Design review of the part built by this model. Coordinates are the model's own, in mm. A direction names the side the tool comes from. Round coordinates to 2 decimals unless told otherwise and drop trailing zeros. Loops run counter-clockwise (first coordinate to the right, second up) from the corner with the lowest first, then second, coordinate; pieces in that order, holes last. Notation, with made-up numbers: (10, 20) - (30, 20) arc R34 cw to (30, 50) - close; hole circle Ø9 at (-36, 42.25). An arc over 180 degrees is marked (long way). Return JSON: item names as keys, results as strings. Group by question number.
from build123d import *

# Parameters (mm, degrees)
SKETCH_1_W          = 50
SKETCH_1_H          = 13
SKETCH_1_R          = 0.5
EXTRUDE_1_DEPTH     = 1.5
SKETCH_3_W          = 7.25
SKETCH_3_H          = 5
EXTRUDE_2_DEPTH     = 4
SKETCH_4_W          = 7.25
SKETCH_4_H          = 5.5
EXTRUDE_3_DEPTH     = 3
CUT_EXTRUDE_1_DEPTH = 7.25
SKETCH_6_W          = 4.302717404
SKETCH_6_H          = 3.6
SKETCH_6_W_2        = 3.2
SKETCH_6_H_2        = 1.274490689
CUT_EXTRUDE_2_DEPTH = 5


with BuildPart() as part:
    # Эскиз1 → Бобышка-Вытянуть1 (new body)
    with BuildSketch(Plane(origin=(0, 0, 0), x_dir=(1, 0, 0), z_dir=(0, 1, 0))):
        with Locations((25, 6.5)):
            Rectangle(SKETCH_1_W, SKETCH_1_H)
        with Locations(Location((1.25, 12, 0), (0, 0, 270))):
            Circle(SKETCH_1_R, mode=Mode.SUBTRACT)
        with Locations(Location((3.75, 12, 0), (0, 0, 270))):
            Circle(SKETCH_1_R, mode=Mode.SUBTRACT)
        with Locations(Location((6.25, 12, 0), (0, 0, 270))):
            Circle(SKETCH_1_R, mode=Mode.SUBTRACT)
        with Locations(Location((8.75, 12, 0), (0, 0, 270))):
            Circle(SKETCH_1_R, mode=Mode.SUBTRACT)
        with Locations(Location((11.25, 12, 0), (0, 0, 270))):
            Circle(SKETCH_1_R, mode=Mode.SUBTRACT)
        with Locations(Location((13.75, 12, 0), (0, 0, 270))):
            Circle(SKETCH_1_R, mode=Mode.SUBTRACT)
        with Locations(Location((16.25, 12, 0), (0, 0, 270))):
            Circle(SKETCH_1_R, mode=Mode.SUBTRACT)
        with Locations(Location((18.75, 12, 0), (0, 0, 270))):
            Circle(SKETCH_1_R, mode=Mode.SUBTRACT)
        with Locations(Location((21.25, 12, 0), (0, 0, 270))):
            Circle(SKETCH_1_R, mode=Mode.SUBTRACT)
        with Locations(Location((23.75, 12, 0), (0, 0, 270))):
            Circle(SKETCH_1_R, mode=Mode.SUBTRACT)
        with Locations(Location((26.25, 12, 0), (0, 0, 270))):
            Circle(SKETCH_1_R, mode=Mode.SUBTRACT)
        with Locations(Location((28.75, 12, 0), (0, 0, 270))):
            Circle(SKETCH_1_R, mode=Mode.SUBTRACT)
        with Locations(Location((31.25, 12, 0), (0, 0, 270))):
            Circle(SKETCH_1_R, mode=Mode.SUBTRACT)
        with Locations(Location((33.75, 12, 0), (0, 0, 270))):
            Circle(SKETCH_1_R, mode=Mode.SUBTRACT)
        with Locations(Location((36.25, 12, 0), (0, 0, 270))):
            Circle(SKETCH_1_R, mode=Mode.SUBTRACT)
        with Locations(Location((3.75, 1, 0), (0, 0, 270))):
            Circle(SKETCH_1_R, mode=Mode.SUBTRACT)
        with Locations(Location((6.25, 1, 0), (0, 0, 270))):
            Circle(SKETCH_1_R, mode=Mode.SUBTRACT)
        with Locations(Location((8.75, 1, 0), (0, 0, 270))):
            Circle(SKETCH_1_R, mode=Mode.SUBTRACT)
        with Locations(Location((11.25, 1, 0), (0, 0, 270))):
            Circle(SKETCH_1_R, mode=Mode.SUBTRACT)
        with Locations(Location((13.75, 1, 0), (0, 0, 270))):
            Circle(SKETCH_1_R, mode=Mode.SUBTRACT)
        with Locations(Location((16.25, 1, 0), (0, 0, 270))):
            Circle(SKETCH_1_R, mode=Mode.SUBTRACT)
        with Locations(Location((18.75, 1, 0), (0, 0, 270))):
            Circle(SKETCH_1_R, mode=Mode.SUBTRACT)
        with Locations(Location((21.25, 1, 0), (0, 0, 270))):
            Circle(SKETCH_1_R, mode=Mode.SUBTRACT)
        with Locations(Location((23.75, 1, 0), (0, 0, 270))):
            Circle(SKETCH_1_R, mode=Mode.SUBTRACT)
        with Locations(Location((26.25, 1, 0), (0, 0, 270))):
            Circle(SKETCH_1_R, mode=Mode.SUBTRACT)
        with Locations(Location((28.75, 1, 0), (0, 0, 270))):
            Circle(SKETCH_1_R, mode=Mode.SUBTRACT)
        with Locations(Location((31.25, 1, 0), (0, 0, 270))):
            Circle(SKETCH_1_R, mode=Mode.SUBTRACT)
        with Locations(Location((33.75, 1, 0), (0, 0, 270))):
            Circle(SKETCH_1_R, mode=Mode.SUBTRACT)
        with Locations(Location((36.25, 1, 0), (0, 0, 270))):
            Circle(SKETCH_1_R, mode=Mode.SUBTRACT)
        with Locations(Location((1.25, 1, 0), (0, 0, 270))):
            Circle(SKETCH_1_R, mode=Mode.SUBTRACT)
        with Locations(Location((38.75, 12, 0), (0, 0, 270))):
            Circle(SKETCH_1_R, mode=Mode.SUBTRACT)
        with Locations(Location((41.25, 12, 0), (0, 0, 270))):
            Circle(SKETCH_1_R, mode=Mode.SUBTRACT)
        with Locations(Location((43.75, 12, 0), (0, 0, 270))):
            Circle(SKETCH_1_R, mode=Mode.SUBTRACT)
        with Locations(Location((46.25, 12, 0), (0, 0, 270))):
            Circle(SKETCH_1_R, mode=Mode.SUBTRACT)
        with Locations(Location((48.75, 12, 0), (0, 0, 270))):
            Circle(SKETCH_1_R, mode=Mode.SUBTRACT)
        with Locations(Location((38.75, 1, 0), (0, 0, 270))):
            Circle(SKETCH_1_R, mode=Mode.SUBTRACT)
        with Locations(Location((41.25, 1, 0), (0, 0, 270))):
            Circle(SKETCH_1_R, mode=Mode.SUBTRACT)
        with Locations(Location((43.75, 1, 0), (0, 0, 270))):
            Circle(SKETCH_1_R, mode=Mode.SUBTRACT)
        with Locations(Location((46.25, 1, 0), (0, 0, 270))):
            Circle(SKETCH_1_R, mode=Mode.SUBTRACT)
        with Locations(Location((48.75, 1, 0), (0, 0, 270))):
            Circle(SKETCH_1_R, mode=Mode.SUBTRACT)
    extrude(amount=EXTRUDE_1_DEPTH)

    # Эскиз3 → Бобышка-Вытянуть2 (add)
    with BuildSketch(Plane(origin=(0, 1.5, 0), x_dir=(1, 0, 0), z_dir=(0, 1, 0))):
        with Locations((47.875, 6.5)):
            Rectangle(SKETCH_3_W, SKETCH_3_H)
    extrude(amount=EXTRUDE_2_DEPTH)

    # Эскиз4 → Бобышка-Вытянуть3 (add)
    with BuildSketch(Plane.XZ):
        with Locations((34.375, -6.75)):
            Rectangle(SKETCH_4_W, SKETCH_4_H)
    extrude(amount=EXTRUDE_3_DEPTH)

    # Эскиз5 → Вырез-Вытянуть1 (cut)
    with BuildSketch(Plane(origin=(51.5, 0, 0), x_dir=(0, 0, -1), z_dir=(1, 0, 0))):
        Polygon((4.148641298, 4.556809932), (4, 4.976937423), (4, 2.023062577), (4.148641298, 2.443190068), (4.148641298, 3.459627547), (4.148641298, 3.540372453), align=None)
        Polygon((9, 2.023062577), (9, 4.976937423), (8.851358702, 4.556809932), (8.851358702, 3.540372453), (8.851358702, 3.459627547), (8.851358702, 2.443190068), align=None)
    extrude(amount=-CUT_EXTRUDE_1_DEPTH, mode=Mode.SUBTRACT)

    # Эскиз6 → Вырез-Вытянуть2 (cut)
    with BuildSketch(Plane(origin=(51.5, 0, 0), x_dir=(0, 0, -1), z_dir=(1, 0, 0))):
        with Locations((6.5, 3.5)):
            Rectangle(SKETCH_6_W, SKETCH_6_H)
        with Locations((6.5, 2.837245345)):
            Rectangle(SKETCH_6_W_2, SKETCH_6_H_2, mode=Mode.SUBTRACT)
    extrude(amount=-CUT_EXTRUDE_2_DEPTH, mode=Mode.SUBTRACT)


solid = part.part
Q1. Tool access review of faces 5 (the flat face through (44.25, 3, -6)), 6 (the flat face through (49, 3, -8.651)), 7 (the cylindrical face through (29.17, 0.74, -0.73)): name each direction out of +Z, -Z, +X, -X, +Y, -Y from which nothing blocks a thin tool from reaching the whole face with its end or side.
Q2. For line 1 (Z direction, x = 41.25, y = 1.1); line 2 (Y direction, x = 23, z = -1.75); line 3 (Z direction, x = 4, y = 1), list the stretches that pass through material, from the lowest coordinate up.
Q3. Insertion check: pin 1 Ø2 at (x, y) = (10, 3.5) entering from +Z; pin 2 Ø2.5 at (x, y) = (34.5, -1.5) entering from +Z; pin 3 Ø1.1 at (x, y) = (46.5, 3.5) entering from -Z; pin 4 Ø1.6 at (x, z) = (48.5, -6.5) entering from -Y. Each pin has a flat end and moves straight along its axis. Give the tip position at first contact, or say it passes through.
Q4. Add section C-C, the plane z = -7. State the section outline as (x, y) points, plus the area to 3 significant figures.
Q5. Add section B-B, the plane x = 16.25. State the section outline as (y, z) points, plus the area to 3 significant figures.
Q6. Draft analysis for pull direction X (two halves, no side actions). For faces 1 (the flat face through (0, 1, -6)), 2 (the cylindrical face through (26.746, 0.74, -12.065)), 3 (the cylindrical face through (21.746, 0.74, -1.065)), 4 (the flat face through (25, 1.5, -7)), state which applies: pulls with the +X half, pulls with the -X half, needs draft (parallel to the pull), parting line crosses it, or undercut.
Q7. Add section A-A, the plane x = 48.75. Give the number of separate pieces and of enclosed holes in the cut face, plus the area to 3 significant figures.
Q8. Add section D-D, the plane y = 4. State the section outline as (x, z) points.
Evaluation:
{
 "1": {"face 5": "+Z, -Z, -X, +Y", "face 6": "+X", "face 7": "+Y, -Y"},
 "2": {"line 1": "-13 to -12.5, -11.5 to -1.5, -0.5 to 0", "line 2": "0 to 1.5", "line 3": "-13 to -12.43, -11.57 to -1.43, -0.57 to 0"},
 "3": {"pin 1": "through", "pin 2": "z = -4", "pin 3": "z = -8.85", "pin 4": "y = 0"},
 "4": {"outline": "(0, 0) - (30.75, 0) - (30.75, -3) - (38, -3) - (38, 0) - (50, 0) - (50, 1.5) - (51.5, 1.5) - (51.5, 1.7) - (46.5, 1.7) - (46.5, 2.2) - (51.5, 2.2) - (51.5, 3.47) - (46.5, 3.47) - (46.5, 5.3) - (51.5, 5.3) - (51.5, 5.5) - (44.25, 5.5) - (44.25, 1.5) - (0, 1.5) - close", "area": "114 mm²"},
 "5": {"outline": "(0, -13) - (1.5, -13) - (1.5, -12.5) - (0, -12.5) - close; (0, -11.5) - (1.5, -11.5) - (1.5, -1.5) - (0, -1.5) - close; (0, -0.5) - (1.5, -0.5) - (1.5, 0) - (0, 0) - close", "area": "16.5 mm²"},
 "6": {"face 1": "pulls with the -X half", "face 2": "undercut", "face 3": "undercut", "face 4": "needs draft"},
 "7": {"separate pieces": "4", "enclosed holes": "1", "area": "24.3 mm²"},
 "8": {"outline": "(44.25, -8.85) - (51.5, -8.85) - (51.5, -8.65) - (46.5, -8.65) - (46.5, -4.35) - (51.5, -4.35) - (51.5, -4.15) - (44.25, -4.15) - close"}
}
